from build123d import *

# Parameters (mm, degrees)
SKETCH_1_W          = 110
SKETCH_1_H          = 38
EXTRUDE_1_DEPTH     = 2
SKETCH_2_W          = 20
SKETCH_2_H          = 2
EXTRUDE_2_DEPTH     = 3
SKETCH_4_W          = 20
SKETCH_4_H          = 2
EXTRUDE_3_DEPTH     = 2
CUT_EXTRUDE_2_DEPTH = 60.270566051
SKETCH_7_R          = 1.5
CUT_EXTRUDE_4_DEPTH = 60.270566051
SKETCH_13_R         = 1.5
CUT_EXTRUDE_6_DEPTH = 60.270566051
FILLET_1_R          = 5
CUT_EXTRUDE_8_DEPTH = 60.270566051


with BuildPart() as part:
    # 草图1 → 凸台-拉伸1 (new body)
    with BuildSketch(Plane(origin=(0, 0, 0), x_dir=(1, 0, 0), z_dir=(0, 1, 0))):
        Rectangle(SKETCH_1_W, SKETCH_1_H)
    extrude(amount=EXTRUDE_1_DEPTH)

    # 草图2 → 凸台-拉伸2 (add)
    with BuildSketch(Plane(origin=(0, 0, -19), x_dir=(-1, 0, 0), z_dir=(0, 0, -1))):
        with Locations((-8, 1)):
            Rectangle(SKETCH_2_W, SKETCH_2_H)
        with Locations((37, 1)):
            Rectangle(SKETCH_2_W, SKETCH_2_H)
    extrude(amount=EXTRUDE_2_DEPTH)

    # 草图4 → 凸台-拉伸3 (add)
    with BuildSketch(Plane.XY.offset(19)):
        with Locations((-15.6, 1)):
            Rectangle(SKETCH_4_W, SKETCH_4_H)
        with Locations((29.4, 1)):
            Rectangle(SKETCH_4_W, SKETCH_4_H)
    extrude(amount=EXTRUDE_3_DEPTH)

    # 草图6 → 切除-拉伸2 (cut, through all)
    with BuildSketch(Plane.XZ):
        with BuildLine():
            Line((53.5, 7.5), (53.5, -7.5))
            ThreePointArc((53.5, -7.5), (52.45, -8.55), (51.4, -7.5))
            Line((51.4, -7.5), (51.4, 7.5))
            ThreePointArc((51.4, 7.5), (52.45, 8.55), (53.5, 7.5))
        make_face()
    extrude(amount=-CUT_EXTRUDE_2_DEPTH, mode=Mode.SUBTRACT)

    # 草图7 → 切除-拉伸4 (cut, through all)
    with BuildSketch(Plane.XZ):
        with Locations(Location((-13, -10, 0), (0, 0, 270))):
            Circle(SKETCH_7_R)
        with Locations(Location((-13, 10, 0), (0, 0, 270))):
            Circle(SKETCH_7_R)
    extrude(amount=-CUT_EXTRUDE_4_DEPTH, mode=Mode.SUBTRACT)

    # 草图13 → 切除-拉伸6 (cut, through all)
    with BuildSketch(Plane(origin=(0, 2, 0), x_dir=(1, 0, 0), z_dir=(0, 1, 0))):
        with Locations((-48.5, 19)):
            Circle(SKETCH_13_R)
        with Locations((-25.5, 19)):
            Circle(SKETCH_13_R)
        with Locations((-3.5, 19)):
            Circle(SKETCH_13_R)
        with Locations((19.5, 19)):
            Circle(SKETCH_13_R)
        with Locations((-27.1, -19)):
            Circle(SKETCH_13_R)
        with Locations((-4.1, -19)):
            Circle(SKETCH_13_R)
        with Locations((17.9, -19)):
            Circle(SKETCH_13_R)
        with Locations((40.9, -19)):
            Circle(SKETCH_13_R)
    extrude(amount=-CUT_EXTRUDE_6_DEPTH, mode=Mode.SUBTRACT)

    # 圆角1
    fillet_1_edges = [part.edges().sort_by_distance(p)[0] for p in [
        (55, 1, 19),
        (-55, 1, 19),
        (-55, 1, -19),
        (55, 1, -19),
    ]]
    fillet(fillet_1_edges, radius=FILLET_1_R - 0.0001)  # a hair under: the kernel refuses the full size

    # 草图12 → 切除-拉伸8 (cut, through all)
    with BuildSketch(Plane(origin=(0, 2, 0), x_dir=(1, 0, 0), z_dir=(0, 1, 0))):
        with BuildLine():
            Line((48, 12), (48, -12))
            ThreePointArc((48, -12), (45, -15), (42, -12))
            Line((42, -12), (42, 12))
            ThreePointArc((42, 12), (45, 15), (48, 12))
        make_face()
        with BuildLine():
            Line((39.5, 12), (39.5, -12))
            ThreePointArc((39.5, -12), (36.5, -15), (33.5, -12))
            Line((33.5, -12), (33.5, 12))
            ThreePointArc((33.5, 12), (36.5, 15), (39.5, 12))
        make_face()
        with BuildLine():
            Line((31, 12), (31, -12))
            ThreePointArc((31, -12), (28, -15), (25, -12))
            Line((25, -12), (25, 12))
            ThreePointArc((25, 12), (28, 15), (31, 12))
        make_face()
        with BuildLine():
            Line((22.5, 12), (22.5, -12))
            ThreePointArc((22.5, -12), (19.5, -15), (16.5, -12))
            Line((16.5, -12), (16.5, 12))
            ThreePointArc((16.5, 12), (19.5, 15), (22.5, 12))
        make_face()
        with BuildLine():
            Line((14, 12), (14, -12))
            ThreePointArc((14, -12), (11, -15), (8, -12))
            Line((8, -12), (8, 12))
            ThreePointArc((8, 12), (11, 15), (14, 12))
        make_face()
        with BuildLine():
            Line((5.5, 12), (5.5, -12))
            ThreePointArc((5.5, -12), (2.5, -15), (-0.5, -12))
            Line((-0.5, -12), (-0.5, 12))
            ThreePointArc((-0.5, 12), (2.5, 15), (5.5, 12))
        make_face()
        with BuildLine():
            Line((-3, 12), (-3, -12))
            ThreePointArc((-3, -12), (-6, -15), (-9, -12))
            Line((-9, -12), (-9, 12))
            ThreePointArc((-9, 12), (-6, 15), (-3, 12))
        make_face()
        with BuildLine():
            Line((-17, 12), (-17, -12))
            ThreePointArc((-17, -12), (-20, -15), (-23, -12))
            Line((-23, -12), (-23, 12))
            ThreePointArc((-23, 12), (-20, 15), (-17, 12))
        make_face()
        with BuildLine():
            Line((-26, 12), (-26, -12))
            ThreePointArc((-26, -12), (-29, -15), (-32, -12))
            Line((-32, -12), (-32, 12))
            ThreePointArc((-32, 12), (-29, 15), (-26, 12))
        make_face()
        with BuildLine():
            Line((-35, 12), (-35, -12))
            ThreePointArc((-35, -12), (-38, -15), (-41, -12))
            Line((-41, -12), (-41, 12))
            ThreePointArc((-41, 12), (-38, 15), (-35, 12))
        make_face()
        with BuildLine():
            Line((-44, 12), (-44, -12))
            ThreePointArc((-44, -12), (-47, -15), (-50, -12))
            Line((-50, -12), (-50, 12))
            ThreePointArc((-50, 12), (-47, 15), (-44, 12))
        make_face()
    extrude(amount=-CUT_EXTRUDE_8_DEPTH, mode=Mode.SUBTRACT)


solid = part.part
Design review of the part built by this model. Coordinates are the model's own, in mm. A direction names the side the tool comes from. Coordinates: 2 decimals unless noted, no trailing zeros. Order: outer loops, then holes, each group sorted by start corner. A loop starts at its lowest first (then second) coordinate and runs counter-clockwise, first axis right, second up.
Item 1: Take a section at C-C, the plane x = 28.5. Write out the cut boundary in (y, z).
Item 2: The part is to be moulded in two halves that separate along X. For faces 4 (the flat face through (-25.6, 1, 20)), 5 (the cylindrical face through (28, 1, -15)), 6 (the flat face through (55, 1, 0)), 7 (the flat face through (-5.6, 1, 20)), say which applies: pulls with the +X half, pulls with the -X half, needs draft (parallel to the pull), parting line crosses it, or undercut.
Item 3: For pin 1 Ø0.6 at (y, z) = (0.5, -20) entering from +X, flat-tipped, find the tip position at first contact; note if it passes through.
Item 4: Take a section at B-B, the plane z = 4.5. Count the separate pieces of the cut face and the enclosed holes in it, then the cut area to 3 significant figures.
Item 5: For line 1 (Z direction, x = -12.5, y = 1.45); line 2 (Z direction, x = 15, y = 1.6); line 3 (Z direction, x = 43, y = 1.75), list the stretches that pass through material, from the lowest coordinate up.
Item 6: For faces 1 (the flat face through (39.4, 1, 20)), 2 (the flat face through (22.5, 1, 0)), 3 (the flat face through (19.4, 1, 20)), list the 3-axis set-ups (+Z, -Z, +X, -X, +Y, -Y) from which the entire face can be reached by the end or side of a thin tool; tool diameter is ignored.
Item 7: Take a section at A-A, the plane x = -20. Write out the cut boundary in (y, z), then the cut area to 3 significant figures.
The answers:
1. outline: (0, -19) - (2, -19) - (2, -14.96) - (0, -14.96) - close; (0, 14.96) - (2, 14.96) - (2, 21) - (0, 21) - close
2. face 4: pulls with the -X half
2. face 5: undercut
2. face 6: pulls with the +X half
2. face 7: undercut
3. pin 1: stops at x = 18
4. separate pieces: 13
4. enclosed holes: 0
4. area: 83.8 mm2
5. line 1: z = -19 to -11.41, -8.59 to 8.59, 11.41 to 21
5. line 2: z = -22 to 19
5. line 3: z = -19 to -14.24, 14.24 to 19
6. face 1: +Z, +X, +Y, -Y
6. face 2: +Y, -Y
6. face 3: +Z, +Y, -Y
7. outline: (0, -19) - (2, -19) - (2, -15) - (0, -15) - close; (0, 15) - (2, 15) - (2, 21) - (0, 21) - close
7. area: 20.0 mm2
